Read the model definition and answer for the solid it produces. Units are mm, in the model's axes. Face numbers are marked on the shaded views. A direction names the side the tool comes from. Coordinates: 2 decimals unless noted, no trailing zeros. Write each loop counter-clockwise with the first axis right and the second up, starting at its lowest first coordinate (ties: lowest second). Pieces come first, ordered by that corner, then holes. Notation, with made-up numbers: (61, 85.5) -> (97, 85.5) arc R13 cw to (97, 100.5) -> close; hole circle Ø10 at (-10.5, 65). An arc over 180 degrees is marked (long way). Answer in a Markdown table with one row per item. Add a question column.
Item 1: Section B-B on x = 0 is taken. Write down the section's boundary in (y, z), then the cut area to 3 significant figures.
Item 2: Section D-D on x = 27.5 is taken. Write down the section's boundary in (y, z), then the cut area to 3 significant figures.
Item 3: Section A-A on z = 4.5 is taken. Write down the section's boundary in (x, y), then the cut area to 3 significant figures.
Item 4: Section C-C on x = 7 is taken. Write down the section's boundary in (y, z).
Item 5: For a pull along Z with two mould halves and no side action, classify the marked faces 1, 2, 3 and 4 as +Z half, -Z half, draft (parallel to the pull), parting line (faces both ways), or undercut.
Item 6: Straight lines are drawn through the part: line 1 (X direction, y = 5.5, z = -28); line 2 (Y direction, x = 0, z = -2); line 3 (Y direction, x = 64, z = -8). For each, find the intervals that lie inside material, in ascending order. Write a range as from..to.
Item 7: Given pin 1 Ø1.5 at (x, z) = (6.5, -26) entering from -Y; pin 2 Ø3 at (x, y) = (37, 0.5) entering from -Z; pin 3 Ø3 at (x, y) = (46, 5.5) entering from -Z; pin 4 Ø5 at (x, z) = (32.5, -11) entering from +Y, each flat-ended and moving along its own axis, determine where each tip first touches the part or whether it passes through.
Item 8: Which of the six approach directions +Z, -Z, +X, -X, +Y, -Y give full straight-line access (tool end or side, diameter ignored) to the marked faces 5, 6, 7, 8 and 9?
```python
from build123d import *

# Parameters (mm, degrees)
BOSS_EXTRUDE1_DEPTH     = 6
SKETCH2_R               = 1.35
CUT_EXTRUDE1_DEPTH      = 39
ESQUISSE1_R             = 4.1
ENL_V_MAT_EXTRU_1_DEPTH = 3


with BuildPart() as part:
    # Sketch1 → Boss-Extrude1 (new body)
    with BuildSketch(Plane(origin=(0, 0, 0), x_dir=(1, 0, 0), z_dir=(0, 1, 0))):
        Polygon((2.5, 0), (0, 0), (0, 25), (2.5, 25), (2.5, 31.5), (-2.5, 31.5), (-2.5, -6.5), (2.5, -6.5), align=None)
        Polygon((0, 25), (0, 0), (2.5, 0), (2.5, 4), (2.5, 21), (2.5, 25), align=None)
        Polygon((32.26, 14.5), (2.5, 25), (2.5, 21), (26.591428571, 12.5), align=None)
        Polygon((26.591428571, 12.5), (32.26, 10.5), (37.928571429, 12.5), (32.26, 14.5), align=None)
        Polygon((32.26, 14.5), (37.928571429, 12.5), (62.02, 21), (62.02, 25), align=None)
        Polygon((2.5, 4), (2.5, 0), (32.26, 10.5), (26.591428571, 12.5), align=None)
        Polygon((32.26, 10.5), (62.02, 0), (62.02, 4), (37.928571429, 12.5), align=None)
        Polygon((62.02, 4), (62.02, 0), (64.52, 0), (64.52, 25), (62.02, 25), (62.02, 21), align=None)
        Polygon((64.52, 0), (62.02, 0), (62.02, -6.5), (67.02, -6.5), (67.02, 31.5), (62.02, 31.5), (62.02, 25), (64.52, 25), align=None)
    extrude(amount=BOSS_EXTRUDE1_DEPTH)

    # Sketch2 → Cut-Extrude1 (cut, through all)
    with BuildSketch(Plane(origin=(0, 0, -31.5), x_dir=(-1, 0, 0), z_dir=(0, 0, -1))):
        with Locations((0, 3)):
            Circle(SKETCH2_R)
        with Locations((-64.52, 3)):
            Circle(SKETCH2_R)
    extrude(amount=-CUT_EXTRUDE1_DEPTH, mode=Mode.SUBTRACT)

    # Esquisse1 → Enlèv. mat.-Extru.1 (cut)
    with BuildSketch(Plane(origin=(0, 6, 0), x_dir=(1, 0, 0), z_dir=(0, 1, 0))):
        with Locations((32.26, 12.5)):
            Circle(ESQUISSE1_R)
    extrude(amount=-ENL_V_MAT_EXTRU_1_DEPTH, mode=Mode.SUBTRACT)


solid = part.part
```
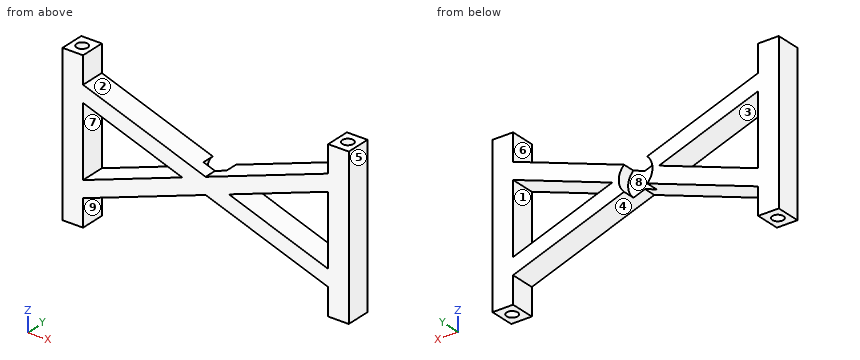
Results below:
| question | item | result |
|---|---|---|
| 1 | outline | (0, -31.5) -> (1.65, -31.5) -> (1.65, 6.5) -> (0, 6.5) -> close; (4.35, -31.5) -> (6, -31.5) -> (6, 6.5) -> (4.35, 6.5) -> close |
| 1 | area | 125 mm2 |
| 2 | outline | (0, -16.18) -> (6, -16.18) -> (6, -8.82) -> (0, -8.82) -> close |
| 2 | area | 44.2 mm2 |
| 3 | outline | (-2.5, 0) -> (2.5, 0) -> (2.5, 6) -> (-2.5, 6) -> close; (62.02, 0) -> (67.02, 0) -> (67.02, 6) -> (62.02, 6) -> close; hole circle Ø2.7 at (0, 3); hole circle Ø2.7 at (64.52, 3) |
| 3 | area | 48.5 mm2 |
| 4 | outline | (0, -23.41) -> (6, -23.41) -> (6, -19.41) -> (0, -19.41) -> close; (0, -5.59) -> (6, -5.59) -> (6, -1.59) -> (0, -1.59) -> close |
| 5 | face 1 | undercut |
| 5 | face 2 | +Z half |
| 5 | face 3 | undercut |
| 5 | face 4 | -Z half |
| 6 | line 1 | x = -2.5..2.5, 62.02..67.02 |
| 6 | line 2 | y = 0..1.65, 4.35..6 |
| 6 | line 3 | y = 0..1.75, 4.25..6 |
| 7 | pin 1 | passes through |
| 7 | pin 2 | stops at z = -16.7 |
| 7 | pin 3 | stops at z = -19.88 |
| 7 | pin 4 | stops at y = 3 |
| 8 | face 5 | +Z, -Z, +X, +Y, -Y |
| 8 | face 6 | +Z, +Y, -Y |
| 8 | face 7 | +Y, -Y |
| 8 | face 8 | +Y |
| 8 | face 9 | -Z, +Y, -Y |
